```python
from build123d import *

# Parameters (mm, degrees)
SKETCH_1_W                       = 120
SKETCH_1_H                       = 20
EXTRUDE_2_DEPTH                  = 2
SM_EDGE_FLANGE_2_STRIP_W         = 12
SM_EDGE_FLANGE_2_STRIP_H         = 2
SM_EDGE_FLANGE_2_STRIP_CUT_DEPTH = 20
SM_EDGE_FLANGE_2_DEPTH           = 20


# Sheet-metal steps are written as plain solids
with BuildPart() as part:
    # Эскиз1 → Бобышка-Вытянуть2 (new body)
    with BuildSketch(Plane.XY):
        with Locations((60, 10)):
            Rectangle(SKETCH_1_W, SKETCH_1_H)
    extrude(amount=EXTRUDE_2_DEPTH)

    # Ребро-кромка2 strip (across the edge) → Ребро-кромка2 strip cut (cut)
    with BuildSketch(Plane(origin=(120, 0, 2), x_dir=(-1, 0, 0), z_dir=(0, 1, 0))):
        with Locations((-2, -1)):
            Rectangle(SM_EDGE_FLANGE_2_STRIP_W, SM_EDGE_FLANGE_2_STRIP_H)
    extrude(amount=SM_EDGE_FLANGE_2_STRIP_CUT_DEPTH, mode=Mode.SUBTRACT)

    # Ребро-кромка2 section (across the edge) → Ребро-кромка2 (add)
    with BuildSketch(Plane(origin=(120, 0, 2), x_dir=(-1, 0, 0), z_dir=(0, 1, 0))):
        with BuildLine():
            Line((0, 2), (0, 118))
            Line((0, 118), (2, 118))
            Line((2, 118), (2, 2))
            ThreePointArc((2, 2), (2.585786438, 0.585786438), (4, 0))
            Line((4, 0), (4, -2))
            ThreePointArc((4, -2), (1.171572875, -0.828427125), (0, 2))
        make_face()
    extrude(amount=SM_EDGE_FLANGE_2_DEPTH)


solid = part.part
```
Check sheet for the modelled part. Datum: model origin and axes. Units: mm. A direction names the side the tool comes from. Give positions to 0.01 mm unless a question says otherwise; leave off trailing zeros. Write each loop counter-clockwise with the first axis right and the second up, starting at its lowest first coordinate (ties: lowest second). Pieces come first, ordered by that corner, then holes.
Item 1: Cross-section at A-A (y = 14.25). Enter the section's corners in (x, z).
Item 2: Cross-section at C-C (z = 104). Enter the section's corners in (x, y).
Item 3: Scan lines: L1, parallel to Z at x = 75, y = 2.25; L2, parallel to X at y = 2, z = 114.5. Record each from-to range of solid material in increasing order.
Item 4: Access from +Z, -Z, +X, -X, +Y, -Y to the whole of each face (thin tool, end or side, straight path). Record for faces 1 (the face through (118.797, 9.86, 1.141)), 2 (the face through (57, 10, 2)).
Item 5: Gauge pin test, flat ends, axial feed: pin 1 (2 mm diameter, centred on y = 9.5, z = 95.5, fed in from -X); pin 2 (5 mm diameter, centred on x = 18.5, y = 10.5, fed in from +Z). Record the tip position at first contact, or that the pin passes through.
Item 6: Cross-section at B-B (x = 27). Enter the section's corners in (y, z), and give its area (3 significant figures).
Report:
1. outline: (0, 0) - (116, 0) arc R4 ccw to (120, 4) - (120, 120) - (118, 120) - (118, 4) arc R2 cw to (116, 2) - (0, 2) - close
2. outline: (118, 0) - (120, 0) - (120, 20) - (118, 20) - close
3. L1: z = 0 to 2
3. L2: x = 118 to 120
4. face 1: -Z, +X, +Y, -Y
4. face 2: +Z, -X, +Y, -Y
5. pin 1: stops at x = 118
5. pin 2: stops at z = 2
6. outline: (0, 0) - (20, 0) - (20, 2) - (0, 2) - close
6. area: 40.0 mm2
